Geometry check sheet. Reference: drawing and pictorial views, mm from the part's lowest x, y, z. Give positions to 0.01 mm unless a question says otherwise; leave off trailing zeros. Order: outer loops, then holes, each group sorted by start corner. A loop starts at its lowest first (then second) coordinate and runs counter-clockwise, first axis right, second up.
Item 1: Material ranges on line 1 along X through (y, z) = (26.5, 1) (1 decimal); line 2 along X through (y, z) = (1, 0.65) (1 decimal); line 3 along Z through (x, y) = (0.95, 15.25), recorded low to high.
Item 2: Gauge pin test, flat end, axial feed: P1, Ø1, axis at x = 1, z = 1, coming from the -Y side (1 decimal). Record the tip position at first contact, or that the pin passes through.
Item 3: Sectioned sample at A-A on y = 7.5. Record the boundary of the cut face in (x, z).
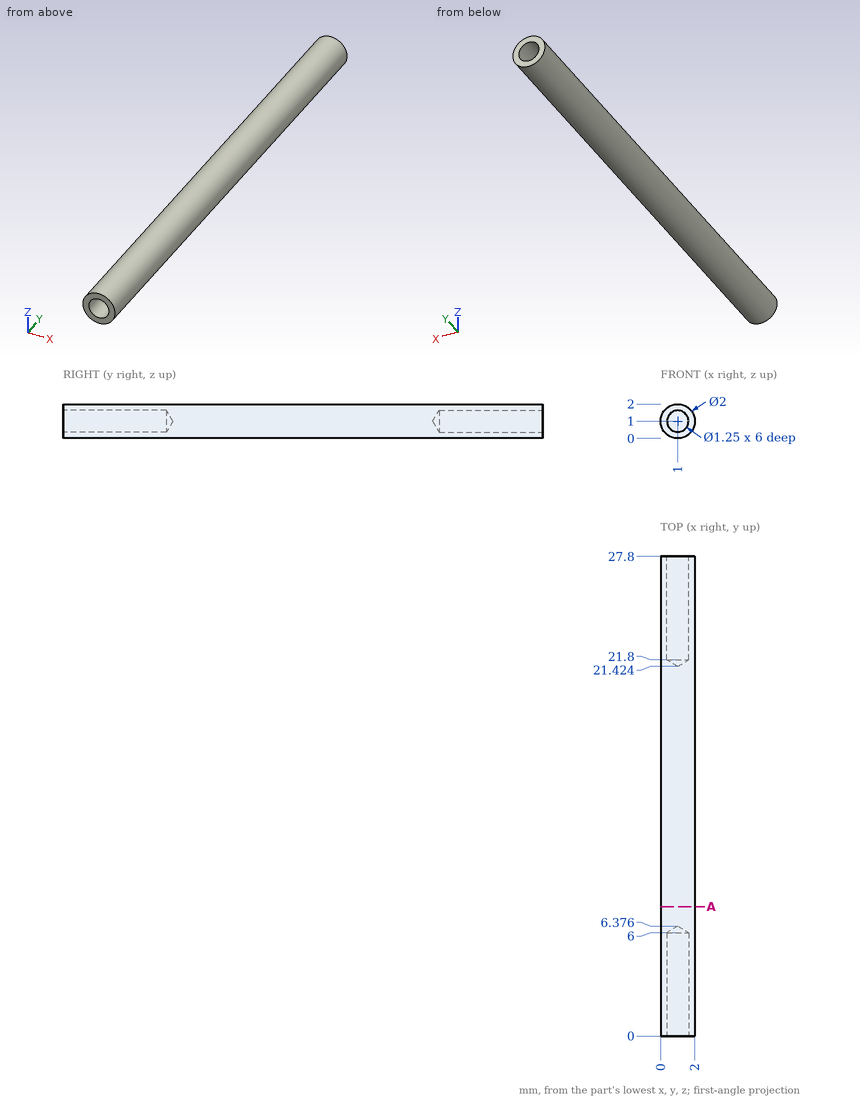
Report:
1. line 1: x = 0 to 0.4, 1.6 to 2
1. line 2: x = 0.1 to 0.5, 1.5 to 1.9
1. line 3: z = 0 to 2
2. P1: stops at y = 6.1
3. outline: circle Ø2 at (1, 1)
